from build123d import *

# Parameters (mm, degrees)
ESQUISSE1_W             = 15
ESQUISSE1_H             = 8.07
BOSS_EXTRU_1_DEPTH      = 2.8
ESQUISSE4_W             = 2.8
ESQUISSE4_H             = 8.07
BOSS_EXTRU_3_DEPTH      = 6.37
BOSS_EXTRU_4_DEPTH      = 15
ESQUISSE6_W             = 2.5
ESQUISSE6_H             = 3.945
ENL_V_MAT_EXTRU_1_DEPTH = 3


with BuildPart() as part:
    # Esquisse1 → Boss.-Extru.1 (new body)
    with BuildSketch(Plane(origin=(0, 0, 0), x_dir=(1, 0, 0), z_dir=(0, 1, 0))):
        with Locations((7.5, 4.035)):
            Rectangle(ESQUISSE1_W, ESQUISSE1_H)
    extrude(amount=BOSS_EXTRU_1_DEPTH)

    # Esquisse4 → Boss.-Extru.3 (add)
    with BuildSketch(Plane(origin=(0, 2.8, 0), x_dir=(1, 0, 0), z_dir=(0, 1, 0))):
        with Locations((16.4, 4.035)):
            Rectangle(ESQUISSE4_W, ESQUISSE4_H)
        with Locations((-1.4, 4.035)):
            Rectangle(ESQUISSE4_W, ESQUISSE4_H)
    extrude(amount=-BOSS_EXTRU_3_DEPTH)

    # Esquisse5 → Boss.-Extru.4 (add)
    with BuildSketch(Plane(origin=(0, 0, 0), x_dir=(0, 0, -1), z_dir=(1, 0, 0))):
        Polygon((8.07, -3.57), (8.07, -1.57), (5.52241552, -1.57), (0, -1.57), (0, -3.57), align=None)
    extrude(amount=BOSS_EXTRU_4_DEPTH)

    # Esquisse6 → Enlèv. mat.-Extru.1 (cut)
    with BuildSketch(Plane.XZ.offset(3.57)):
        with Locations((7.655, -5.581368507)):
            Rectangle(ESQUISSE6_W, ESQUISSE6_H)
    extrude(amount=-ENL_V_MAT_EXTRU_1_DEPTH, mode=Mode.SUBTRACT)


solid = part.part
Input: part model. Units: mm. Frame: model coordinates. A direction names the side the tool comes from. Round coordinates to 2 decimals unless told otherwise and drop trailing zeros. Order: outer loops, then holes, each group sorted by start corner. A loop starts at its lowest first (then second) coordinate and runs counter-clockwise, first axis right, second up. Notation, with made-up numbers: (53, 63.25) - (102, 63.25) arc R10 ccw to (102, 76.25) - close; hole circle Ø5 at (13.25, -21.75). An arc over 180 degrees is marked (long way). Use a Markdown table: item, result.
1. Section C-C on x = 8. Return the cut outline in (y, z), then the cut area to 3 significant figures.
Evaluation:
| item | result |
|---|---|
| outline | (-3.57, -8.07) - (-1.57, -8.07) - (-1.57, -7.55) - (-3.57, -7.55) - close; (-3.57, -3.61) - (-1.57, -3.61) - (-1.57, 0) - (-3.57, 0) - close; (0, -8.07) - (2.8, -8.07) - (2.8, 0) - (0, 0) - close |
| area | 30.8 mm^2 |
2. Mould query, pull axis Z, two halves, no side actions, for faces 1 (the face through (7, 0, -4)), 2 (the face through (7.4, 0.4, 0)), 3 (the face through (6.405, -3, -6)). Classes: +Z half, -Z half, draft (parallel to the pull), parting line (faces both ways), or undercut.
Evaluation:
| item | result |
|---|---|
| face 1 | draft |
| face 2 | +Z half |
| face 3 | undercut |
3. Section A-A on x = 2.5. Return the cut outline in (y, z).
Evaluation:
| item | result |
|---|---|
| outline | (-3.57, -8.07) - (-1.57, -8.07) - (-1.57, 0) - (-3.57, 0) - close; (0, -8.07) - (2.8, -8.07) - (2.8, 0) - (0, 0) - close |
4. Section D-D on z = -5.75. Return the cut outline in (x, y) (3 decimals).
Evaluation:
| item | result |
|---|---|
| outline | (-2.8, -3.57) - (6.405, -3.57) - (6.405, -1.57) - (0, -1.57) - (0, 0) - (15, 0) - (15, -1.57) - (8.905, -1.57) - (8.905, -3.57) - (17.8, -3.57) - (17.8, 2.8) - (-2.8, 2.8) - close |
5. Access query for faces 4 (the face through (8, -3, -7.554)), 5 (the face through (7, -1.57, -3)), 6 (the face through (7, 2.8, -4)). Directions: +Z, -Z, +X, -X, +Y, -Y. A direction counts if a zero-diameter tool reaches every point of the face in a straight line with its end or side. Return the directions, or none.
Evaluation:
| item | result |
|---|---|
| face 4 | -Y |
| face 5 | +Z, -Z |
| face 6 | +Z, -Z, +X, -X, +Y |
6. Material intervals for probe 1 along Y at (x, z) = (11, -0.5); probe 2 along X at (y, z) = (-2.75, -5.5) (3 decimals); probe 3 along X at (y, z) = (-1, -1.25), sorted ascending.
Evaluation:
| item | result |
|---|---|
| probe 1 | -3.57 to -1.57, 0 to 2.8 |
| probe 2 | -2.8 to 6.405, 8.905 to 17.8 |
| probe 3 | -2.8 to 0, 15 to 17.8 |
7. Section B-B on y = -1. Return the cut outline in (x, z), then the cut area to 3 significant figures.
Evaluation:
| item | result |
|---|---|
| outline | (-2.8, -8.07) - (0, -8.07) - (0, 0) - (-2.8, 0) - close; (15, -8.07) - (17.8, -8.07) - (17.8, 0) - (15, 0) - close |
| area | 45.2 mm^2 |
